Geometry: final body of the model. Coordinates: model frame, mm. Coordinates: 2 decimals unless noted, no trailing zeros. Order: outer loops, then holes, each group sorted by start corner. A loop starts at its lowest first (then second) coordinate and runs counter-clockwise, first axis right, second up. Notation, with made-up numbers: M 26.25,48 L 75.25,48 A14 ccw 75.25,75 Z; hole C 28.25,29 d9. An arc over 180 degrees is marked long. Write item = value, one per line. Start each with the question number.
```python
from build123d import *

# Parameters (mm, degrees)
SKETCH_1_R               = 45
SKETCH_1_R_2             = 35
EXTRUDE_1_DEPTH          = 3
EXTRUDE_2_DEPTH          = 3
SKETCH_3_R               = 1.5
CUT_EXTRUDE_1_DEPTH      = 3
PATTERN_CIRCULAR_1_COUNT = 14
FILLET_1_R               = 3
EXTRUDE_3_DEPTH          = 3
FILLET_2_R               = 3
FILLET_3_R               = 1
FILLET_4_R               = 3


with BuildPart() as part:
    # Эскиз1 → Бобышка-Вытянуть1 (new body)
    with BuildSketch(Plane(origin=(0, 0, 0), x_dir=(1, 0, 0), z_dir=(0, 1, 0))):
        with Locations(Location((0, 0, 0), (0, 0, 270))):
            Circle(SKETCH_1_R)
        with Locations(Location((0, 0, 0), (0, 0, 270))):
            Circle(SKETCH_1_R_2, mode=Mode.SUBTRACT)
    extrude(amount=EXTRUDE_1_DEPTH)

    # Эскиз2 → Бобышка-Вытянуть2 (add)
    with BuildSketch(Plane(origin=(0, 0, 0), x_dir=(1, 0, 0), z_dir=(0, 1, 0))):
        with BuildLine():
            ThreePointArc((-34.391132578, 6.5), (-34.847450698, 3.264227303), (-35, 0))
            Line((-35, 0), (35, 0))
            ThreePointArc((35, 0), (34.847450698, 3.264227303), (34.391132578, 6.5))
            Line((34.391132578, 6.5), (-34.391132578, 6.5))
        make_face()
        with BuildLine():
            Line((35, 0), (-35, 0))
            ThreePointArc((-35, 0), (-34.847450698, -3.264227303), (-34.391132578, -6.5))
            Line((-34.391132578, -6.5), (34.391132578, -6.5))
            ThreePointArc((34.391132578, -6.5), (34.847450698, -3.264227303), (35, 0))
        make_face()
    extrude(amount=EXTRUDE_2_DEPTH)

    # Эскиз3 → Вырез-Вытянуть1 (cut)
    with BuildSketch(Plane(origin=(0, 3, 0), x_dir=(1, 0, 0), z_dir=(0, 1, 0))):
        with Locations(Location((0, 40, 0), (0, 0, 270))):
            Circle(SKETCH_3_R)
    cut_extrude_1 = extrude(amount=-CUT_EXTRUDE_1_DEPTH, mode=Mode.SUBTRACT)

    # Круговой массив1: Вырез-Вытянуть1 ×14 about axis
    pattern_circular_1_axis = Axis((0, 0, 0), (0, 1, 0))
    for i in range(1, PATTERN_CIRCULAR_1_COUNT):
        add(cut_extrude_1.rotate(pattern_circular_1_axis, i * 360 / PATTERN_CIRCULAR_1_COUNT), mode=Mode.SUBTRACT)

    # Скругление1
    fillet_1_edges = [part.edges().sort_by_distance(p)[0] for p in [
        (-34.391132578, 1.5, -6.5),
        (-34.391132578, 1.5, 6.5),
        (34.391132578, 1.5, 6.5),
        (34.391132578, 1.5, -6.5),
    ]]
    fillet(fillet_1_edges, radius=FILLET_1_R)

    # Эскиз4 → Бобышка-Вытянуть3 (add)
    with BuildSketch(Plane(origin=(0, 0, 0), x_dir=(1, 0, 0), z_dir=(0, 1, 0))):
        with BuildLine():
            Line((-3.5, 6.5), (-3.5, 34.824560299))
            ThreePointArc((-3.5, 34.824560299), (-7.551905138, 34.175557476), (-11.5, 33.056769352))
            Line((-11.5, 33.056769352), (-11.5, 6.5))
            Line((-11.5, 6.5), (-3.5, 6.5))
        make_face()
        with BuildLine():
            Line((3.5, 6.5), (3.5, 34.824560299))
            ThreePointArc((3.5, 34.824560299), (7.551905138, 34.175557476), (11.5, 33.056769352))
            Line((11.5, 33.056769352), (11.5, 6.5))
            Line((11.5, 6.5), (3.5, 6.5))
        make_face()
    extrude_3 = extrude(amount=EXTRUDE_3_DEPTH)

    # Скругление2
    fillet_2_edges = [part.edges().sort_by_distance(p)[0] for p in [
        (-11.5, 1.5, -6.5),
        (-3.5, 1.5, -34.824560299),
        (-11.5, 1.5, -33.056769352),
        (11.5, 1.5, -6.5),
        (11.5, 1.5, -33.056769352),
        (3.5, 1.5, -34.824560299),
    ]]
    fillet(fillet_2_edges, radius=FILLET_2_R)

    # Зеркальное отражение1: Бобышка-Вытянуть3 across plane
    add(extrude_3.mirror(Plane.XY))

    # Скругление3
    fillet_3_edges = [part.edges().sort_by_distance(p)[0] for p in [
        (-3.5, 1.5, -6.5),
        (3.5, 1.5, -6.5),
        (-3.5, 1.5, 6.5),
        (3.5, 1.5, 6.5),
    ]]
    fillet(fillet_3_edges, radius=FILLET_3_R)

    # Скругление4
    fillet_4_edges = [part.edges().sort_by_distance(p)[0] for p in [
        (-11.5, 1.5, 6.5),
        (-11.5, 1.5, 33.056769352),
        (-3.5, 1.5, 34.824560299),
        (11.5, 1.5, 6.5),
        (3.5, 1.5, 34.824560299),
        (11.5, 1.5, 33.056769352),
    ]]
    fillet(fillet_4_edges, radius=FILLET_4_R)


solid = part.part
```
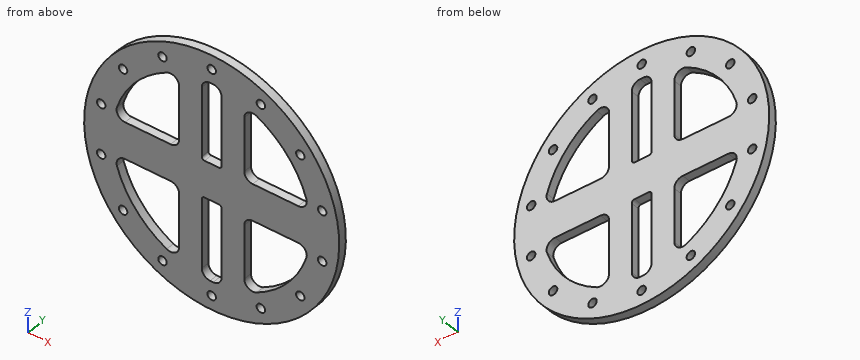
Item 1: Section query A-A on x = 26. Output: boundary loops of the cut face in (y, z), and give its area (3 significant figures).
Item 2: Section query C-C on z = 40. Output: boundary loops of the cut face in (x, y).
Item 3: Section query B-B on z = -12.5. Output: boundary loops of the cut face in (x, y).
Item 4: First-contact query: pin 1 (0.9 mm diameter, centred on x = 23, y = 1, fed in from -Z); pin 2 (2.5 mm diameter, centred on x = 31.27, z = 24.94, fed in from +Y); pin 3 (1 mm diameter, centred on y = 1, z = -8.5, fed in from +X); pin 4 (0.9 mm diameter, centred on y = 2, z = -21.5, fed in from +X). Flat tips, straight axial feed; report the tip coordinate or a pass-through.
Item 5: Section query D-D on z = 17.5. Output: boundary loops of the cut face in (x, y).
Item 6: Material intervals for probe 1 along X at (y, z) = (0.2, 10.5); probe 2 along Z at (x, y) = (-14, 1.6); probe 3 along X at (y, z) = (2.15, 17.5), sorted ascending. Write a range as [from, to].
Ans:
q1.outline = M 0,-36.73 L 3,-36.73 L 3,-23.43 L 0,-23.43 Z; M 0,-6.5 L 3,-6.5 L 3,6.5 L 0,6.5 Z; M 0,23.43 L 3,23.43 L 3,36.73 L 0,36.73 Z
q1.area = 119 mm^2
q2.outline = M -20.62,0 L -1.5,0 L -1.5,3 L -20.62,3 Z; M 1.5,0 L 20.62,0 L 20.62,3 L 1.5,3 Z
q3.outline = M -43.23,0 L -32.69,0 L -32.69,3 L -43.23,3 Z; M -11.5,0 L -3.5,0 L -3.5,3 L -11.5,3 Z; M 3.5,0 L 11.5,0 L 11.5,3 L 3.5,3 Z; M 32.69,0 L 43.23,0 L 43.23,3 L 32.69,3 Z
q4.pin_1 = -38.94
q4.pin_2 = through
q4.pin_3 = 44.28
q4.pin_4 = 39.77
q5.outline = M -41.46,0 L -30.31,0 L -30.31,3 L -41.46,3 Z; M -11.5,0 L -3.5,0 L -3.5,3 L -11.5,3 Z; M 3.5,0 L 11.5,0 L 11.5,3 L 3.5,3 Z; M 30.31,0 L 41.46,0 L 41.46,3 L 30.31,3 Z
q6.probe_1 = [-43.76, -33.39], [-11.5, -3.5], [3.5, 11.5], [33.39, 43.76]
q6.probe_2 = [-42.77, -31.48], [-6.54, 6.54], [31.48, 42.77]
q6.probe_3 = [-41.46, -30.31], [-11.5, -3.5], [3.5, 11.5], [30.31, 41.46]
